```python
from build123d import *

# Parameters (mm, degrees)
F0_W     = 40
F0_H     = 215
F1_DEPTH = 15
F2_W     = 39.6
F2_H     = 29.6
F3_DEPTH = 214.8
F5_DEPTH = 62.4
F6_R     = 3


with BuildPart() as f1:
    # F0 (on Front) → F1 (new body, symmetric)
    with BuildSketch(Plane.XZ):
        Rectangle(F0_W, F0_H)
    extrude(amount=F1_DEPTH, both=True)

    # F2 (on face) → F3 (cut)
    with BuildSketch(Plane.XY.offset(107.5)):
        Rectangle(F2_W, F2_H)
    extrude(amount=-F3_DEPTH, mode=Mode.SUBTRACT)

    # F4 (on face) → F5 (cut, symmetric)
    with BuildSketch(Plane(origin=(-20, 0, 0), x_dir=(0, -1, 0), z_dir=(-1, 0, 0))):
        with BuildLine():
            Line((5, 107.5), (-5, 107.5))
            ThreePointArc((-5, 107.5), (0, 102.5), (5, 107.5))
        make_face()
    extrude(amount=F5_DEPTH, both=True, mode=Mode.SUBTRACT)

    # F6
    f6_edges = [f1.edges().sort_by_distance(p)[0] for p in [
        (19.9, -5, 107.5),
        (-19.9, -5, 107.5),
        (19.9, 5, 107.5),
        (-19.9, 5, 107.5),
    ]]
    fillet(f6_edges, radius=F6_R)


solid = f1.part
```
Input: part model. Units: mm. Frame: model coordinates. A direction names the side the tool comes from. Coordinates: 2 decimals unless noted, no trailing zeros. Order: outer loops, then holes, each group sorted by start corner. A loop starts at its lowest first (then second) coordinate and runs counter-clockwise, first axis right, second up. Notation, with made-up numbers: (32.5, 32.5) - (64.5, 32.5) arc R26 cw to (64.5, 69.5) - close; hole circle Ø3 at (71.25, 28). An arc over 180 degrees is marked (long way). Put each result on its own line as item: value.
1. Reachability of faces 4 (the face through (-20, 0, -2)), 5 (the face through (-19.8, 0, 2)) from +Z, -Z, +X, -X, +Y, -Y: full face, straight path, thin tool, end or side. Return the list, or none.
Report:
face 4: +Z, -Z, -X, +Y, -Y
face 5: +Z
2. Line query: line 1 along X through (y, z) = (8, 10); line 2 along Y through (x, z) = (17.5, -74); line 3 along Z through (x, y) = (3.5, -6). Output: solid intervals per line, ascending.
Report:
line 1: x = -20 to -19.8, 19.8 to 20
line 2: y = -15 to -14.8, 14.8 to 15
line 3: z = -107.5 to -107.3
3. Draft query along Y for faces 1 (the face through (0, -15, 2)), 2 (the face through (0, 0, -107.5)), 3 (the face through (0, -14.8, 2)). Return one class per face: pulls with the +Y half, pulls with the -Y half, needs draft (parallel to the pull), parting line crosses it, or undercut.
Report:
face 1: pulls with the -Y half
face 2: needs draft
face 3: undercut
4. Cut plane A-A on x = -7.5. Return the cut outline in (y, z).
Report:
outline: (-15, -107.5) - (15, -107.5) - (15, 107.5) - (14.8, 107.5) - (14.8, -107.3) - (-14.8, -107.3) - (-14.8, 107.5) - (-15, 107.5) - close
5. Cut plane C-C on y = -2.5. Return the cut outline in (x, z).
Report:
outline: (-20, -107.5) - (20, -107.5) - (20, 103.17) - (19.8, 103.17) - (19.8, -107.3) - (-19.8, -107.3) - (-19.8, 103.17) - (-20, 103.17) - close
6. Cut plane B-B on z = 70.5. Return the cut outline in (x, y), then the cut area to 3 significant figures.
Report:
outline: (-20, -15) - (20, -15) - (20, 15) - (-20, 15) - close; hole (-19.8, -14.8) - (19.8, -14.8) - (19.8, 14.8) - (-19.8, 14.8) - close
area: 27.8 mm2
7. Contact query for a flat-ended pin moving along its axis: pin 1 Ø6 at (x, y) = (-0.5, 0.5) entering from +Z. Output: stop coordinate, or through.
Report:
pin 1: stops at z = -107.3
